from build123d import *

# Parameters (mm, degrees)
BOSS_EXTRUDE1_DEPTH     = 598
SKETCH2_W               = 90
SKETCH2_H               = 15
BOSS_EXTRUDE2_DEPTH     = 39
CUT_EXTRUDE1_DEPTH      = 458.203414552
CUT_EXTRUDE1_DEPTH_BACK = 458.203414552
SKETCH3_R               = 7.875


with BuildPart() as part:
    # Sketch1 → Boss-Extrude1 (new body)
    with BuildSketch(Plane(origin=(0, 0, 0), x_dir=(1, 0, 0), z_dir=(0, 1, 0))):
        with BuildLine():
            Line((-76, 0), (76, 0))
            ThreePointArc((76, 0), (54.45181356, 55.029972187), (0, 78))
            ThreePointArc((0, 78), (-53.858440233, 54.45181356), (-76, 0))
        make_face()
    extrude(amount=BOSS_EXTRUDE1_DEPTH)

    # Sketch2 → Boss-Extrude2 (add)
    with BuildSketch(Plane.XY):
        with Locations((0, 446.94016831)):
            Rectangle(SKETCH2_W, SKETCH2_H)
        with Locations((0, 161.460515061)):
            Rectangle(SKETCH2_W, SKETCH2_H)
    extrude(amount=BOSS_EXTRUDE2_DEPTH)

    # Sketch3 → Cut-Extrude1 (cut, two sides: drawn at the far end of the back side and taken through both)
    with BuildSketch(Plane(origin=(0, 153.960515061, 0), x_dir=(-1, 0, 0), z_dir=(0, -1, 0)).offset(-CUT_EXTRUDE1_DEPTH_BACK)):
        with Locations(Location((0, -22.983942377, 0), (0, 0, 90))):
            Circle(SKETCH3_R)
    extrude(amount=CUT_EXTRUDE1_DEPTH + CUT_EXTRUDE1_DEPTH_BACK, mode=Mode.SUBTRACT)


solid = part.part
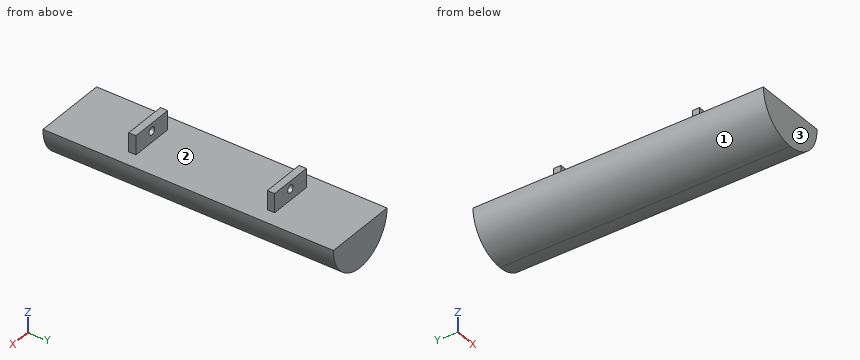
Read the model definition and answer for the solid it produces. Units are mm, in the model's axes. Face numbers are marked on the shaded views. Coordinates: 2 decimals unless noted, no trailing zeros. Write each loop counter-clockwise with the first axis right and the second up, starting at its lowest first coordinate (ties: lowest second). Pieces come first, ordered by that corner, then holes. Notation, with made-up numbers: (-40, 74.25) -> (-21, 74.25) arc R23 ccw to (-21, 97.25) -> close; hole circle Ø10 at (38, 33.5). An arc over 180 degrees is marked (long way). Return JSON: item names as keys, results as strings.
(1) The part is cut by section B-B on z = -20. Give the vertices of the cut face in (x, y), then the cut area to 3 significant figures.
Answers below:
{"outline": "(-73.39, 0) -> (73.86, 0) -> (73.86, 598) -> (-73.39, 598) -> close", "area": "88,100 mm^2"}
(2) Each of these flat-tipped pins is pushed along its axis until it touches: P1, Ø2, axis at x = -28.5, z = 7, coming from the +Y side; P2, Ø7.5, axis at y = 445.5, z = 15.5, coming from the +X side; P3, Ø5, axis at x = 40, z = 8, coming from the -Y side. Where does it stop, or does it pass through?
Answers below:
{"P1": "y = 454.44", "P2": "x = 45", "P3": "y = 153.96"}
(3) The part is cut by section D-D on x = -14. Give the vertices of the cut face in (y, z), then the cut area to 3 significant figures.
Answers below:
{"outline": "(0, -76.36) -> (598, -76.36) -> (598, 0) -> (454.44, 0) -> (454.44, 39) -> (439.44, 39) -> (439.44, 0) -> (168.96, 0) -> (168.96, 39) -> (153.96, 39) -> (153.96, 0) -> (0, 0) -> close", "area": "46,800 mm^2"}
(4) Consider line 1 along Z through (x, y) = (0, 448.25); line 2 along Y through (x, z) = (44, 4); line 3 along X through (y, z) = (450.5, 29.5). Determine where each line is inside the solid, lowest interval first. Write a range as from..to.
Answers below:
{"line 1": "-78..15.11, 30.86..39", "line 2": "153.96..168.96, 439.44..454.44", "line 3": "-45..-4.42, 4.42..45"}
(5) For a pull along Y with two mould halves and no side action, classify the marked faces 1, 2 and 3 as pulls with the +Y half, pulls with the -Y half, needs draft (parallel to the pull), parting line crosses it, or undercut.
Answers below:
{"face 1": "needs draft", "face 2": "undercut", "face 3": "pulls with the -Y half"}
(6) The part is cut by section A-A on x = 16. Give the vertices of the cut face in (y, z).
Answers below:
{"outline": "(0, -76.3) -> (598, -76.3) -> (598, 0) -> (454.44, 0) -> (454.44, 39) -> (439.44, 39) -> (439.44, 0) -> (168.96, 0) -> (168.96, 39) -> (153.96, 39) -> (153.96, 0) -> (0, 0) -> close"}
(7) The part is cut by section C-C on y = 518.5. Give the vertices of the cut face in (x, z).
Answers below:
{"outline": "(-76, 0) arc R78.03 ccw to (0, -78) arc R76.03 ccw to (76, 0) -> close"}
